Could you check a few things on this drawing? It's one solid part, dimensions in mm from its lowest x, y, z. Give positions to 0.01 mm unless a question says otherwise; leave off trailing zeros. Order: outer loops, then holes, each group sorted by start corner. A loop starts at its lowest first (then second) coordinate and runs counter-clockwise, first axis right, second up.
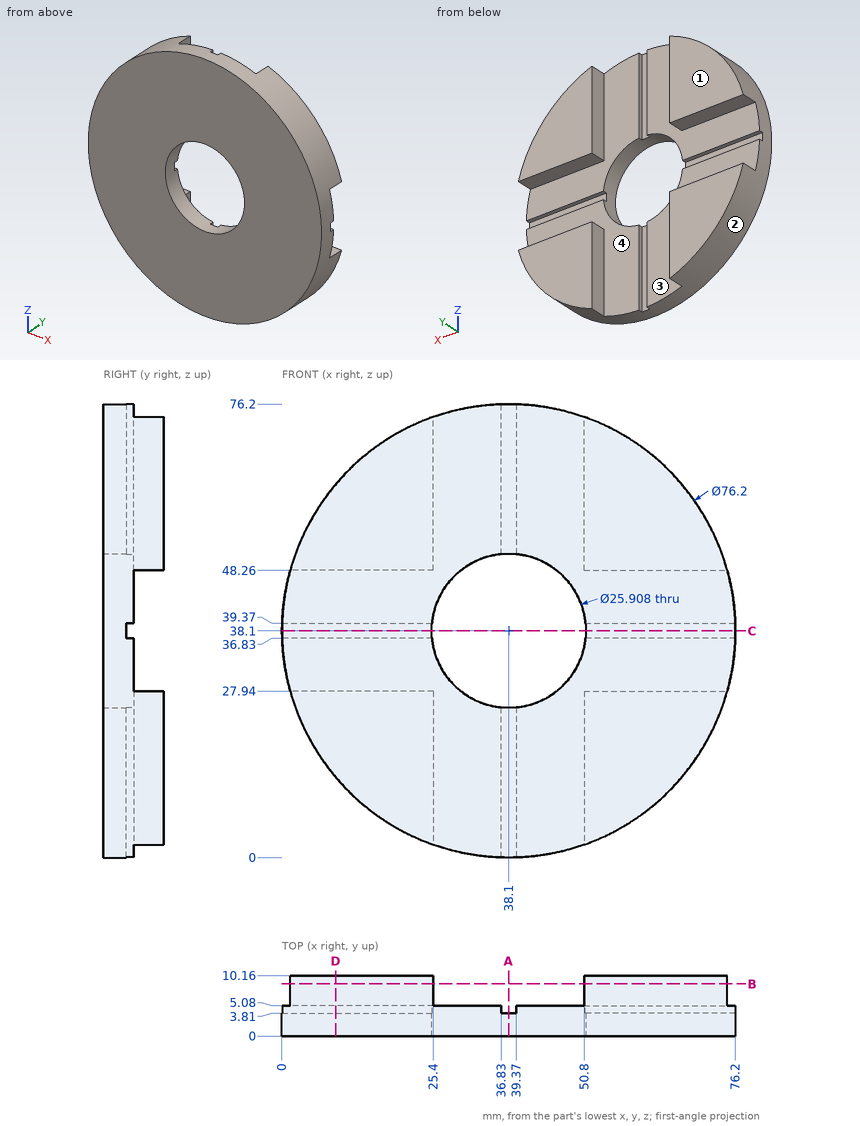
Q1. I'm going to push flat-ended pins straight in: P1, Ø1.5, axis at x = 9, y = 7.5, coming from the +Z side; P2, Ø1, axis at x = 31, y = 7.5, coming from the -Z side; P3, Ø0.6, axis at y = 4.5, z = 69.5, coming from the +X side; P4, Ø1.5, axis at y = 4.5, z = 29.5, coming from the +X side. Where does each tip first touch, or does it pass through?
Filled sheet:
P1: stops at z = 63.55
P2: passes through
P3: stops at x = 60.11
P4: stops at x = 75.38
Q2. I need wall thicknesses on L1, parallel to X at y = 2.7, z = 38.1; L2, parallel to Y at x = 72.5, z = 46. Which ranges of each line are inside material? Lowest first, please.
Filled sheet:
L1: x = 0 to 25.15, 51.05 to 76.2
L2: y = 0 to 5.08
Q3. If we section it at A-A on x = 38.1: List the corners of the cut face in (y, z) for me, plus the area to 3 significant figures.
Filled sheet:
outline: (0, 0) - (3.81, 0) - (3.81, 25.15) - (0, 25.15) - close; (0, 51.05) - (3.81, 51.05) - (3.81, 76.2) - (0, 76.2) - close
area: 192 mm2
Q4. If we section it at C-C on z = 38.1: List the corners of the cut face in (x, y) for me, plus the area to 3 significant figures.
Filled sheet:
outline: (0, 0) - (25.15, 0) - (25.15, 3.81) - (0, 3.81) - close; (51.05, 0) - (76.2, 0) - (76.2, 3.81) - (51.05, 3.81) - close
area: 192 mm2
Q5. Thinking about a two-plate mould opening in Z: for the marked faces 1, 2, 3 and 4, which applies, released by +Z, released by -Z, zero draft, split by the parting line, or undercut?
Filled sheet:
face 1: zero draft
face 2: split by the parting line
face 3: undercut
face 4: undercut
Q6. If we section it at D-D on x = 9: List the corners of the cut face in (y, z) for me, plus the area to 3 significant figures.
Filled sheet:
outline: (0, 13.51) - (10.16, 13.51) - (10.16, 27.94) - (5.08, 27.94) - (5.08, 36.83) - (3.81, 36.83) - (3.81, 39.37) - (5.08, 39.37) - (5.08, 48.26) - (10.16, 48.26) - (10.16, 62.69) - (0, 62.69) - close
area: 393 mm2
Q7. If we section it at B-B on y = 8.75: List the corners of the cut face in (x, z) for me, plus the area to 3 significant figures.
Filled sheet:
outline: (1.38, 27.94) arc R38.1 ccw to (25.4, 2.18) - (25.4, 27.94) - close; (1.38, 48.26) - (25.4, 48.26) - (25.4, 74.02) arc R38.1 ccw to start; (50.8, 2.18) arc R38.1 ccw to (74.82, 27.94) - (50.8, 27.94) - close; (50.8, 48.26) - (74.82, 48.26) arc R38.1 ccw to (50.8, 74.02) - close
area: 1,650 mm2
